For this review, take the finished solid that the model builds, in its own axes (mm). Face numbers are marked on the shaded views. A direction names the side the tool comes from. Round coordinates to 2 decimals unless told otherwise and drop trailing zeros. Write each loop counter-clockwise with the first axis right and the second up, starting at its lowest first coordinate (ties: lowest second). Pieces come first, ordered by that corner, then holes. Notation, with made-up numbers: (48.5, 28) - (76.5, 28) arc R18 ccw to (76.5, 53) - close; hole circle Ø9 at (51, 17). An arc over 180 degrees is marked (long way). Answer in a Markdown table with one row per item. Add a question column.
from build123d import *

# Parameters (mm, degrees)
F0_W     = 34
F0_H     = 35
F1_DEPTH = 9
F3_DEPTH = 56.9500997663
F4_W     = 6
F4_H     = 9


with BuildPart() as f1:
    # F0 (on Top) → F1 (new body)
    with BuildSketch(Plane.XY):
        Rectangle(F0_W, F0_H)
    extrude(amount=F1_DEPTH)

    # F2 (on face) → F3 (cut)
    with BuildSketch(Plane.XZ.offset(17.5)):
        Polygon((-7, 1), (-7, 0), (0, 0), (0, 7), (-15, 7), (-15, 1), align=None)
        Polygon((0, 7), (0, 0), (7, 0), (7, 1), (15, 1), (15, 7), align=None)
    extrude(amount=-F3_DEPTH, mode=Mode.SUBTRACT)

    # F4 (on Front) → F6 (revolve)
    with BuildSketch(Plane.XZ):
        with Locations((3, 13.5)):
            Rectangle(F4_W, F4_H)
        with BuildLine():
            Line((0, 18), (6, 18))
            ThreePointArc((6, 18), (4.2426406871, 22.2426406871), (0, 24))
            Line((0, 24), (0, 18))
        make_face()
    revolve(axis=Axis((0, 0, 0), (0, 0, 1)))


solid = f1.part
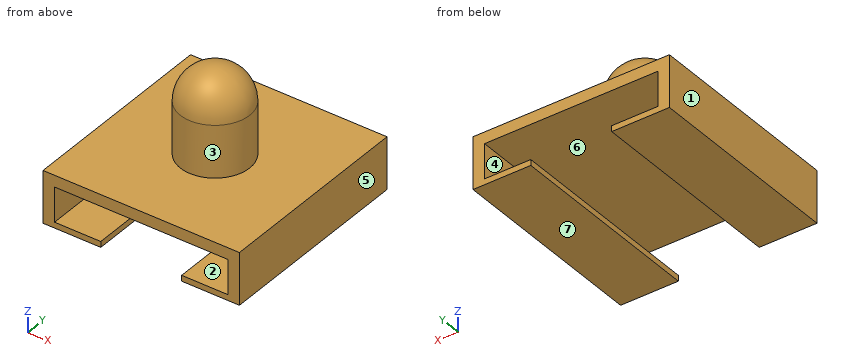
Q1. Draft analysis for pull direction Z (two halves, no side actions). For the marked faces 4, 5, 6 and 7, state which applies: released by +Z, released by -Z, zero draft, split by the parting line, or undercut.
Q2. Add section C-C on x = 0. State the section outline as (y, z) points.
Q3. Add section D-D on y = 0. State the section outline as (x, z) points.
Q4. Insertion check: pin 1 Ø10 at (x, y) = (-6, 5) entering from +Z; pin 2 Ø1 at (x, y) = (-3.5, -2) entering from -Z; pin 3 Ø1 at (x, y) = (-9, 12.5) entering from +Z. Each pin has a flat end and moves straight along its axis. Give the tip position at first contact, or say it passes through.
Q5. To check wall thickness, follow probe 1 along X at (y, z) = (-9, 1.75); probe 2 along Z at (x, y) = (-9.5, -12.5); probe 3 along Z at (x, y) = (-2.5, -14). State the ranges of each line that lie inside material, in increasing order.
Q6. Add section A-A on z = 5.5. State the section outline as (x, y) points, then the cut area to 3 significant figures.
Q7. Tool access review of the marked faces 1, 2 and 3: name each direction out of +Z, -Z, +X, -X, +Y, -Y from which nothing blocks a thin tool from reaching the whole face with its end or side.
Q8. Add section B-B on y = 7. State the section outline as (x, z) points.
Answer sheet:
| question | item | result |
|---|---|---|
| 1 | face 4 | undercut |
| 1 | face 5 | zero draft |
| 1 | face 6 | undercut |
| 1 | face 7 | released by -Z |
| 2 | outline | (-17.5, 7) - (17.5, 7) - (17.5, 9) - (6, 9) - (6, 18) arc R6 ccw to (-6, 18) - (-6, 9) - (-17.5, 9) - close |
| 3 | outline | (-17, 0) - (-7, 0) - (-7, 1) - (-15, 1) - (-15, 7) - (15, 7) - (15, 1) - (7, 1) - (7, 0) - (17, 0) - (17, 9) - (6, 9) - (6, 18) arc R6 ccw to (-6, 18) - (-6, 9) - (-17, 9) - close |
| 4 | pin 1 | stops at z = 23.3 |
| 4 | pin 2 | stops at z = 7 |
| 4 | pin 3 | stops at z = 9 |
| 5 | probe 1 | x = -17 to -15, 15 to 17 |
| 5 | probe 2 | z = 0 to 1, 7 to 9 |
| 5 | probe 3 | z = 7 to 9 |
| 6 | outline | (-17, -17.5) - (-15, -17.5) - (-15, 17.5) - (-17, 17.5) - close; (15, -17.5) - (17, -17.5) - (17, 17.5) - (15, 17.5) - close |
| 6 | area | 140 mm² |
| 7 | face 1 | +Z, -Z, -X, +Y, -Y |
| 7 | face 2 | +Y, -Y |
| 7 | face 3 | +Z |
| 8 | outline | (-17, 0) - (-7, 0) - (-7, 1) - (-15, 1) - (-15, 7) - (15, 7) - (15, 1) - (7, 1) - (7, 0) - (17, 0) - (17, 9) - (-17, 9) - close |
